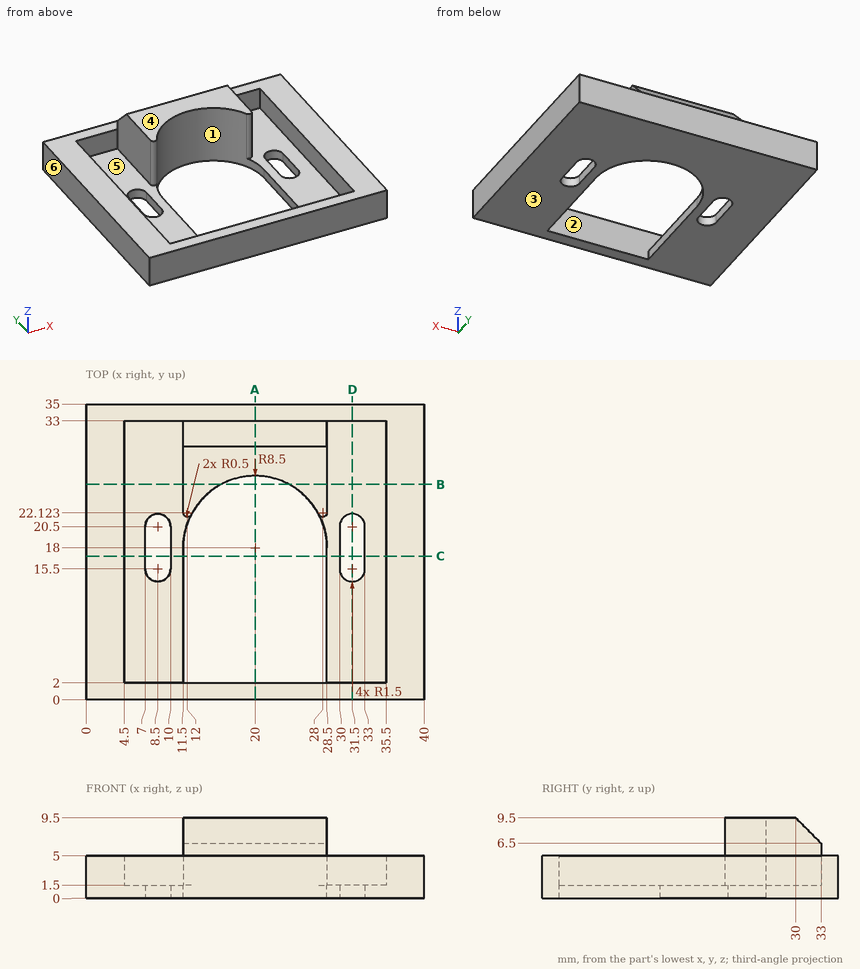
Job drawing, mm, ordinate dimensions from the low corner. One solid piece. A direction names the side the tool comes from. Round coordinates to 2 decimals unless told otherwise and drop trailing zeros. Loops run counter-clockwise (first coordinate to the right, second up) from the corner with the lowest first, then second, coordinate; pieces in that order, holes last.
(1) Which spindle directions (+Z, -Z, +X, -X, +Y, -Y) get a long thin tool onto all of the face, cutting with end or side? Do the marked faces 1, 2 and 3. Say none if no direction does.
(2) Drop flat-ended pins along their axis: pin 1 (8.5 mm diameter, centred on x = 31, y = 11, fed in from +Z); pin 2 (1.2 mm diameter, centred on x = 22, z = 6, fed in from +Y). Give the stop position or say it passes through.
(3) Two-plate mould, pull along X, no slides. Class the marked faces 4, 5 and 6: +X half, -X half, draft (parallel to the pull), parting line (faces both ways), or undercut.
(4) Wall check: line 1 along X through (y, z) = (27, 4.5); line 2 along X through (y, z) = (9, 1.75); line 3 along Z through (x, y) = (36.5, 10). Give the ranges that are in metal, low to high.
(5) Cut at D-D (x = 31.5). Give the cut face in (y, z).
(6) Cut at B-B (y = 25.5). Give the cut face in (x, z).
(7) Cut at C-C (y = 17). Give the cut face in (x, z), plus the area to 3 significant figures.
(8) Cut at A-A (x = 20). Give the cut face in (y, z).
Findings below:
1. face 1: +Z, -Z
1. face 2: +Z
1. face 3: -Z, +X, -X, +Y, -Y
2. pin 1: stops at z = 1.5
2. pin 2: stops at y = 33
3. face 4: draft
3. face 5: undercut
3. face 6: -X half
4. line 1: x = 0 to 4.5, 11.5 to 28.5, 35.5 to 40
4. line 2: x = 0 to 4.5, 35.5 to 40
4. line 3: z = 0 to 5
5. outline: (0, 0) - (14, 0) - (14, 1.5) - (2, 1.5) - (2, 5) - (0, 5) - close; (22, 0) - (35, 0) - (35, 5) - (33, 5) - (33, 1.5) - (22, 1.5) - close
6. outline: (0, 0) - (16, 0) - (16, 9.5) - (11.5, 9.5) - (11.5, 1.5) - (4.5, 1.5) - (4.5, 5) - (0, 5) - close; (24, 0) - (40, 0) - (40, 5) - (35.5, 5) - (35.5, 1.5) - (28.5, 1.5) - (28.5, 9.5) - (24, 9.5) - close
7. outline: (0, 0) - (7, 0) - (7, 1.5) - (4.5, 1.5) - (4.5, 5) - (0, 5) - close; (10, 0) - (11.5, 0) - (11.5, 1.5) - (10, 1.5) - close; (28.5, 0) - (30, 0) - (30, 1.5) - (28.5, 1.5) - close; (33, 0) - (40, 0) - (40, 5) - (35.5, 5) - (35.5, 1.5) - (33, 1.5) - close
7. area: 57.0 mm2
8. outline: (0, 0) - (2, 0) - (2, 5) - (0, 5) - close; (26.5, 0) - (35, 0) - (35, 5) - (33, 5) - (33, 6.5) - (30, 9.5) - (26.5, 9.5) - close
